Verification items for the finished model (mm, model axes). A direction names the side the tool comes from. Give positions to 0.01 mm unless a question says otherwise; leave off trailing zeros. Order: outer loops, then holes, each group sorted by start corner. A loop starts at its lowest first (then second) coordinate and runs counter-clockwise, first axis right, second up.
(1) Mould release check, pull along Y, two halves, no side actions. Record for faces 6 (the face through (26.58, 52.44, 2.03)), 7 (the face through (19, 43, 1)), 8 (the face through (20, 21, 0)): pulls with the +Y half, pulls with the -Y half, needs draft (parallel to the pull), parting line crosses it, or undercut.
(2) Sectioned sample at C-C on x = 9. Record the cut outline in (y, z), plus the area to 3 significant figures.
(3) Gauge pin test, flat ends, axial feed: pin 1 (1.2 mm diameter, centred on y = 36.5, z = 2.5, fed in from -X); pin 2 (2 mm diameter, centred on x = 17.5, y = 37.5, fed in from -Z); pin 3 (5.5 mm diameter, centred on y = 22, z = 24.5, fed in from -X); pin 4 (4 mm diameter, centred on x = 10, z = 47.5, fed in from +Y). Record the tip position at first contact, or that the pin passes through.
(4) Sectioned sample at A-A on x = 31.5. Record the cut outline in (y, z), plus the area to 3 significant figures.
(5) Sectioned sample at B-B on y = 24. Record the cut outline in (x, z), plus the area to 3 significant figures.
(6) Sectioned sample at D-D on z = 13.5. Record the cut outline in (x, y).
(7) Access from +Z, -Z, +X, -X, +Y, -Y to the whole of each face (thin tool, end or side, straight path). Record for faces 1 (the face through (35, 30, 2)), 2 (the face through (5.5, 23, 34)), 3 (the face through (18.5, 23, 34)), 4 (the face through (20, 35, 3)), 5 (the face through (35, 23, 2)).
(8) Scan lines: L1, parallel to Z at x = 17.5, y = 45; L2, parallel to Z at x = 24, y = 47; L3, parallel to Y at x = 16, z = 44. Record each from-to range of solid material in increasing order.
Autodesk Fusion 360 part; units mm, degrees
sketch "スケッチ1" plane through (0, 0, 0) normal (0, 0, 1) x (1, 0, 0)
  line L0 (0, 0) -> (40, 0)
  line L1 (40, 0) -> (40, 30)
  line L2 (40, 30) -> (0, 30)
  line L3 (0, 30) -> (0, 0)
  line L4 (6, 21) -> (18, 21)
  line L5 (18, 21) -> (18, 25)
  line L6 (18, 25) -> (6, 25)
  line L7 (6, 25) -> (6, 21)
  line L8 (21, 20) -> (35, 20)
  line L9 (35, 20) -> (35, 26)
  line L10 (35, 26) -> (21, 26)
  line L11 (21, 26) -> (21, 20)
  dimension "d1" = 30
extrude "押し出し1" add sketch "スケッチ1" along normal blind 4
sketch "スケッチ2" plane through (0, 0, 4) normal (0, 0, 1) x (-1, 0, 0)
  line L0 (-6, -21) -> (-6, -25)
  line L1 (-6, -25) -> (-18, -25)
  line L2 (-18, -25) -> (-18, -21)
  line L3 (-18, -21) -> (-6, -21)
  line L4 (-21, -20) -> (-21, -26)
  line L5 (-21, -26) -> (-35, -26)
  line L6 (-35, -26) -> (-35, -20)
  line L7 (-35, -20) -> (-21, -20)
  line L8 (0, -30) -> (0, 0)
  line L9 (0, 0) -> (-40, 0)
  line L10 (-40, 0) -> (-40, -30)
  line L11 (-40, -30) -> (0, -30)
sketch "スケッチ3" plane through (0, 0, 0) normal (0, 0, -1) x (1, 0, 0)
  line L0 (6, -25) -> (6, -21)
  line L1 (6, -21) -> (18, -21)
  line L2 (18, -21) -> (18, -25)
  line L3 (18, -25) -> (6, -25)
  line L4 (21, -26) -> (21, -20)
  line L5 (21, -20) -> (35, -20)
  line L6 (35, -20) -> (35, -26)
  line L7 (35, -26) -> (21, -26)
  line L8 (0, 0) -> (0, -30)
  line L9 (0, -30) -> (40, -30)
  line L10 (40, -30) -> (40, 0)
  line L11 (40, 0) -> (0, 0)
  line L12 (19, -21) -> (5, -21)
  line L13 (5, -21) -> (5, -26)
  line L14 (5, -26) -> (19, -26)
  line L15 (19, -26) -> (19, -21)
extrude "押し出し2" cut sketch "スケッチ3" against normal blind 1 contours L0 L2 L3 L12 L13 L14 L15
sketch "スケッチ4" plane through (0, 0, 0) normal (0, 0, -1) x (1, 0, 0)
  line L0 (0, 0) -> (0, -30)
  line L1 (0, -30) -> (40, -30)
  line L2 (40, -30) -> (40, 0)
  line L3 (40, 0) -> (0, 0)
  line L4 (21, -26) -> (21, -20)
  line L5 (21, -20) -> (35, -20)
  line L6 (35, -20) -> (35, -26)
  line L7 (35, -26) -> (21, -26)
  line L8 (5, -21) -> (19, -21)
  line L9 (19, -21) -> (19, -26)
  line L10 (19, -26) -> (5, -26)
  line L11 (5, -26) -> (5, -21)
sketch "スケッチ5" plane through (0, 0, 0) normal (0, 0, -1) x (1, 0, 0)
  line L0 (11, -30) -> (29, -30)
  line L1 (29, -30) -> (29, -55)
  line L2 (29, -55) -> (11, -55)
  line L3 (11, -55) -> (11, -30)
  line L4 (19, -48) -> (19, -37)
  line L5 (21, -48) -> (21, -37)
  circle A0 centre (20, -48) radius 1
  circle A1 centre (20, -37) radius 1
extrude "押し出し3" add sketch "スケッチ5" against normal blind 4
fillet "フィレット1" radius 8.5 2 edges at (11, 55, 2) (29, 55, 2)
sketch "スケッチ6" plane through (0, 0, 4) normal (0, 0, 1) x (-1, 0, 0)
  line L0 (-19, -21) -> (-5, -21)
  line L1 (-5, -21) -> (-5, -26)
  line L2 (-5, -26) -> (-19, -26)
  line L3 (-19, -26) -> (-19, -21)
extrude "押し出し4" cut sketch "スケッチ6" against normal blind 2
extrude "押し出し5" add sketch "スケッチ4" against normal blind 1 contours L8 L9 L10 L11
extrude "押し出し6" cut sketch "スケッチ2" against normal blind 200 contours L0 L1 L2 L3
sketch "スケッチ7" plane through (0, 0, 4) normal (0, 0, 1) x (-1, 0, 0)
  line L0 (-19, -21) -> (-5, -21)
  line L1 (-5, -21) -> (-5, -26)
  line L2 (-5, -26) -> (-19, -26)
  line L3 (-19, -26) -> (-19, -21)
  arc A0 (-29, -46.5) -> (-20.5, -55) centre (-20.5, -46.5) ccw
  line L4 (-20.5, -55) -> (-19.5, -55)
  arc A1 (-19.5, -55) -> (-11, -46.5) centre (-19.5, -46.5) ccw
  line L5 (-11, -46.5) -> (-11, -30)
  line L6 (-11, -30) -> (0, -30)
  line L7 (0, -30) -> (0, 0)
  line L8 (0, 0) -> (-40, 0)
  line L9 (-40, 0) -> (-40, -30)
  line L10 (-40, -30) -> (-29, -30)
  line L11 (-29, -30) -> (-29, -46.5)
  arc A2 (-21, -48) -> (-19, -48) centre (-20, -48) ccw
  line L12 (-21, -48) -> (-21, -37)
  arc A3 (-19, -37) -> (-21, -37) centre (-20, -37) ccw
  line L13 (-19, -37) -> (-19, -48)
  line L14 (-21, -20) -> (-21, -26)
  line L15 (-21, -26) -> (-35, -26)
  line L16 (-35, -26) -> (-35, -20)
  line L17 (-35, -20) -> (-21, -20)
  line L18 (-17, -50) -> (-23, -50)
  line L19 (-23, -50) -> (-23, -35)
  line L20 (-23, -35) -> (-17, -35)
  line L21 (-17, -35) -> (-17, -50)
extrude "押し出し7" cut sketch "スケッチ7" against normal blind 2.2 contours L18 L19 L20 L21
sketch "スケッチ8" plane through (0, 0, 0) normal (0, 0, -1) x (1, 0, 0)
  line L0 (18, -25) -> (6, -25)
  line L1 (6, -25) -> (6, -21)
  line L2 (6, -21) -> (18, -21)
  line L3 (18, -21) -> (18, -25)
  arc A0 (19, -48) -> (21, -48) centre (20, -48) ccw
  line L4 (19, -48) -> (19, -37)
  arc A1 (21, -37) -> (19, -37) centre (20, -37) ccw
  line L5 (21, -37) -> (21, -48)
  arc A2 (20.5, -55) -> (29, -46.5) centre (20.5, -46.5) ccw
  line L6 (29, -46.5) -> (29, -30)
  line L7 (29, -30) -> (40, -30)
  line L8 (40, -30) -> (40, 0)
  line L9 (40, 0) -> (0, 0)
  line L10 (0, 0) -> (0, -30)
  line L11 (0, -30) -> (11, -30)
  line L12 (11, -30) -> (11, -46.5)
  arc A3 (11, -46.5) -> (19.5, -55) centre (19.5, -46.5) ccw
  line L13 (19.5, -55) -> (20.5, -55)
  line L14 (21, -26) -> (21, -20)
  line L15 (21, -20) -> (35, -20)
  line L16 (35, -20) -> (35, -26)
  line L17 (35, -26) -> (21, -26)
  line L18 (18.5, -25.5) -> (5.5, -25.5)
  line L19 (5.5, -25.5) -> (5.5, -20.5)
  line L20 (5.5, -20.5) -> (18.5, -20.5)
  line L21 (18.5, -20.5) -> (18.5, -25.5)
  line L22 (5, -26) -> (19, -26)
  line L23 (19, -26) -> (19, -21)
  line L24 (19, -21) -> (5, -21)
  line L25 (5, -21) -> (5, -26)
extrude "押し出し8" add 1 faces at (10, 25.6667, 2) along direction (0, 0, 1) blind 2
extrude "押し出し9" add sketch "スケッチ8" against normal blind 65 contours L0 L1 L3 L18 L19 L21 L24 | L0 L1 L2 L3 L24 | L2 L19 L20 L21 L24
Ans:
1. face 6: pulls with the +Y half
1. face 7: undercut
1. face 8: needs draft
2. outline: (0, 0) - (30, 0) - (30, 4) - (25.5, 4) - (25.5, 65) - (20.5, 65) - (20.5, 4) - (0, 4) - close
2. area: 425 mm2
3. pin 1: stops at x = 11
3. pin 2: stops at z = 0
3. pin 3: stops at x = 5.5
3. pin 4: stops at y = 25.5
4. outline: (0, 0) - (20, 0) - (20, 4) - (0, 4) - close; (26, 0) - (30, 0) - (30, 4) - (26, 4) - close
4. area: 96.0 mm2
5. outline: (0, 0) - (21, 0) - (21, 4) - (18.5, 4) - (18.5, 65) - (5.5, 65) - (5.5, 4) - (0, 4) - close; (35, 0) - (40, 0) - (40, 4) - (35, 4) - close
5. area: 897 mm2
6. outline: (5.5, 20.5) - (18.5, 20.5) - (18.5, 25.5) - (5.5, 25.5) - close
7. face 1: +Z, -Z, +X, +Y
7. face 2: +Z, -X, +Y, -Y
7. face 3: +Z, +X, +Y, -Y
7. face 4: +Z
7. face 5: +Z, -Z
8. L1: z = 0 to 1.8
8. L2: z = 0 to 4
8. L3: y = 20.5 to 25.5
